```python
from build123d import *

# Parameters (mm, degrees)
BOSS_EXTRUDE1_DEPTH     = 9
CUT_EXTRUDE2_DEPTH      = 12.895377253
SKETCH6_W               = 3
SKETCH6_H               = 6
BOSS_EXTRUDE3_DEPTH     = 5
SKETCH7_W               = 3
SKETCH7_H               = 3
REVOLVE1_ANGLE          = 180
SKETCH9_R               = 1.45
CUT_EXTRUDE3_DEPTH      = 5
SKETCH10_W              = 3
SKETCH10_H              = 6
BOSS_EXTRUDE4_DEPTH     = 5
SKETCH12_W              = 3
SKETCH12_H              = 3
REVOLVE2_ANGLE          = 180
SKETCH14_R              = 1.45
CUT_EXTRUDE4_DEPTH      = 5
CUT_EXTRUDE5_DEPTH      = 19.694919096
CUT_EXTRUDE5_DEPTH_BACK = 19.694919096


with BuildPart() as part:
    # Sketch2 → Boss-Extrude1 (new, symmetric)
    with BuildSketch(Plane(origin=(0, 0, 0), x_dir=(1, 0, 0), z_dir=(0, 1, 0))):
        Polygon((-3, 5.5), (3, 5.5), (5.5, 3), (5.5, -3), (3, -5.5), (-3, -5.5), (-5.5, -3), (-5.5, 3), align=None)
    extrude(amount=BOSS_EXTRUDE1_DEPTH, both=True)

    # Sketch5 → Cut-Extrude2 (cut, symmetric)
    with BuildSketch(Plane(origin=(0, 0, 0), x_dir=(0, 0, -1), z_dir=(1, 0, 0))):
        Polygon((0, 9), (0, 8.99), (5.5, 3.49), (5.5, 9), align=None)
    cut_extrude2 = extrude(amount=CUT_EXTRUDE2_DEPTH, both=True, mode=Mode.SUBTRACT)

    # Mirror3: Cut-Extrude2 across plane
    add(cut_extrude2.mirror(Plane.ZX), mode=Mode.SUBTRACT)

    # Sketch6 → Boss-Extrude3 (add, symmetric)
    with BuildSketch(Plane.XZ.offset(9)):
        with Locations((-4, 0)):
            Rectangle(SKETCH6_W, SKETCH6_H)
    boss_extrude3 = extrude(amount=BOSS_EXTRUDE3_DEPTH, both=True)

    # Sketch7 → Revolve1 (revolve)
    with BuildSketch(Plane.XZ.offset(14)):
        with Locations((-4, 1.5)):
            Rectangle(SKETCH7_W, SKETCH7_H)
    revolve1 = revolve(axis=Axis((-5.5, -14, 0), (1, 0, 0)), revolution_arc=REVOLVE1_ANGLE)

    # Sketch9 → Cut-Extrude3 (cut, symmetric)
    with BuildSketch(Plane.ZY.offset(5.5)):
        with Locations((0, -14)):
            Circle(SKETCH9_R)
    cut_extrude3 = extrude(amount=CUT_EXTRUDE3_DEPTH, both=True, mode=Mode.SUBTRACT)

    # Mirror5: Boss-Extrude3, Revolve1, Cut-Extrude3 across plane
    add(boss_extrude3.mirror(Plane(origin=(0, 0, 0), x_dir=(0, 0, 1), z_dir=(1, 0, 0))))
    add(revolve1.mirror(Plane(origin=(0, 0, 0), x_dir=(0, 0, 1), z_dir=(1, 0, 0))))
    add(cut_extrude3.mirror(Plane(origin=(0, 0, 0), x_dir=(0, 0, 1), z_dir=(1, 0, 0))), mode=Mode.SUBTRACT)

    # Sketch10 → Boss-Extrude4 (add, symmetric)
    with BuildSketch(Plane(origin=(0, 9, 0), x_dir=(1, 0, 0), z_dir=(0, 1, 0))):
        Rectangle(SKETCH10_W, SKETCH10_H)
    extrude(amount=BOSS_EXTRUDE4_DEPTH, both=True)

    # Sketch12 → Revolve2 (revolve)
    with BuildSketch(Plane(origin=(0, 14, 0), x_dir=(1, 0, 0), z_dir=(0, 1, 0))):
        with Locations((0, 1.5)):
            Rectangle(SKETCH12_W, SKETCH12_H)
    revolve(axis=Axis((-1.5, 14, 0), (1, 0, 0)), revolution_arc=REVOLVE2_ANGLE)

    # Sketch14 → Cut-Extrude4 (cut, symmetric)
    with BuildSketch(Plane.ZY.offset(1.5)):
        with Locations((0, 14)):
            Circle(SKETCH14_R)
    extrude(amount=CUT_EXTRUDE4_DEPTH, both=True, mode=Mode.SUBTRACT)

    # Sketch15 → Cut-Extrude5 (cut, two sides: drawn at the far end of the back side and taken through both)
    with BuildSketch(Plane(origin=(0, 0, 0), x_dir=(1, 0, 0), z_dir=(0, 1, 0)).offset(-CUT_EXTRUDE5_DEPTH_BACK)):
        Polygon((0, 5), (-1, 4), (-1, 3), (1, 3), (1, 4), align=None)
        Polygon((1, -4), (0, -3), (-1, -4), (-1, -5), (1, -5), align=None)
    extrude(amount=CUT_EXTRUDE5_DEPTH + CUT_EXTRUDE5_DEPTH_BACK, mode=Mode.SUBTRACT)


solid = part.part
```
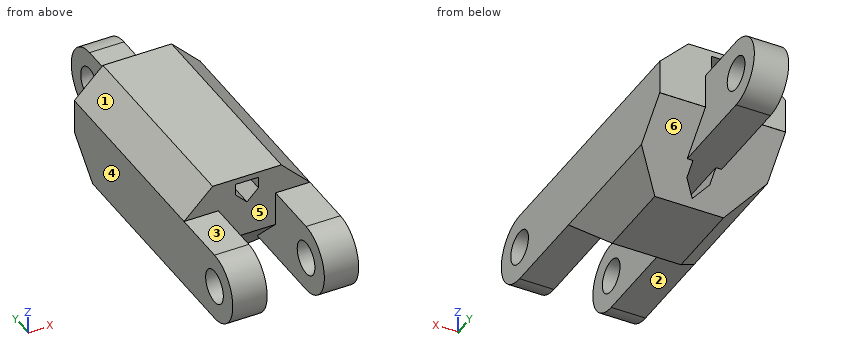
Verification items for the finished model (mm, model axes). Face numbers are marked on the shaded views. A direction names the side the tool comes from. Coordinates: 2 decimals unless noted, no trailing zeros. Order: outer loops, then holes, each group sorted by start corner. A loop starts at its lowest first (then second) coordinate and runs counter-clockwise, first axis right, second up. Notation, with made-up numbers: (-6, -34) -> (14, -34) arc R22 cw to (14, 0) -> close; hole circle Ø8 at (43.5, 43). An arc over 180 degrees is marked (long way). Answer as CSV lines item,"result". Start each with the question number.
1) Gauge pin test, flat ends, axial feed: pin 1 Ø1.5 at (x, y) = (0.5, 12.5) entering from +Z; pin 2 Ø0.9 at (x, y) = (3.5, -10.5) entering from -Z; pin 3 Ø4 at (x, z) = (1.5, 3) entering from -Y. Record the tip position at first contact, or that the pin passes through.
2) Cross-section at C-C, the plane y = -2. Record the boundary of the cut face in (x, z), then the cut area to 4 significant figures.
3) Cross-section at D-D, the plane z = 2.25. Record the boundary of the cut face in (x, y), then the cut area to 3 significant figures.
4) Material ranges on L1, parallel to X at y = -8, z = -2.5; L2, parallel to Z at x = 0.5, y = 4; L3, parallel to Y at x = -3.5, z = 3.75, recorded low to high. Write a range as [from, to].
5) Set-up check for the marked faces 1, 2 and 3: record each of +Z, -Z, +X, -X, +Y, -Y from which the full face is reachable in a straight line by a thin tool's end or side.
6) Release check for a two-part mould opening along X. For the marked faces 4, 5 and 6 record: released by +X, released by -X, zero draft, split by the parting line, or undercut.
7) Cross-section at B-B, the plane y = -8. Record the boundary of the cut face in (x, z), then the cut area to 3 significant figures.
Conclusion:
1,pin 1,"stops at z = 3"
1,pin 2,"stops at z = -3"
1,pin 3,"stops at y = -16.72"
2,outline,"(-5.5, -3) -> (-3, -5.5) -> (3, -5.5) -> (5.5, -3) -> (5.5, 3) -> (3, 5.5) -> (-3, 5.5) -> (-5.5, 3) -> close; hole (-1, -4) -> (0, -5) -> (1, -4) -> (1, -3) -> (-1, -3) -> close; hole (-1, 4) -> (0, 3) -> (1, 4) -> (1, 5) -> (-1, 5) -> close"
2,area,"102.5 mm²"
3,outline,"(-5.5, -15.98) -> (-2.5, -15.98) -> (-2.5, -9) -> (2.5, -9) -> (2.5, -15.98) -> (5.5, -15.98) -> (5.5, 9) -> (1.5, 9) -> (1.5, 15.98) -> (-1.5, 15.98) -> (-1.5, 9) -> (-5.5, 9) -> close"
3,area,"261 mm²"
4,L1,"x = [-5.5, -2.5], [2.5, 5.5]"
4,L2,"z = [-4.99, -4.5], [-3, 3.5], [5, 5.5]"
4,L3,"y = [-9, 9]"
5,face 1,"+Z, -X, +Y, -Y"
5,face 2,"-Z, +X, -X, -Y"
5,face 3,"+Z, +X, -X, -Y"
6,face 4,"released by -X"
6,face 5,"undercut"
6,face 6,"zero draft"
7,outline,"(-5.5, -3) -> (-2.5, -3) -> (-2.5, -0.99) -> (2.5, -0.99) -> (2.5, -3) -> (5.5, -3) -> (5.5, 3) -> (3, 5.5) -> (-3, 5.5) -> (-5.5, 3) -> close; hole (-1, 4) -> (0, 3) -> (1, 4) -> (1, 5) -> (-1, 5) -> close"
7,area,"74.2 mm²"
